Can you work these out from the model? Positions are in its coordinate system, mm. A direction names the side the tool comes from. Give positions to 0.01 mm unless a question says otherwise; leave off trailing zeros. Loops run counter-clockwise (first coordinate to the right, second up) from the corner with the lowest first, then second, coordinate; pieces in that order, holes last. Notation, with made-up numbers: (48, -36.5) - (88, -36.5) arc R11 cw to (88, -28.5) - close; hole circle Ø9 at (-2, -38.75). An arc over 180 degrees is marked (long way). Answer as a JSON object with one key per item and string values. Group by question number.
Item 1: Thinking about a two-plate mould opening in X: for faces 1 (the cylindrical face through (16.3, 7.21, 2.35)), 2 (the flat face through (66.65, 22, 2)), 3 (the flat face through (33, 44.45, 2)), which applies, pulls with the +X half, pulls with the -X half, needs draft (parallel to the pull), parting line crosses it, or undercut?
Item 2: Which directions (+Z, -Z, +X, -X, +Y, -Y) give clear straight access to the entire face, cutting with the end or side of a thin tool? Please do faces 4 (the cylindrical face through (43.9, 25.6, 3.7)), 5 (the cylindrical face through (47.3, 7.21, 2.35)).
Item 3: Will this pin go through, and if not, where does the flat tip stop? pin 1 (18 mm diameter, centred on x = 34.5, y = 23, fed in from +Z).
Item 4: Suppose I cut it at C-C on z = 1.1. Write out the boundary of the cut face in (x, y) (3 decimals).
Item 5: Suppose I cut it at A-A on y = 23. Write out the boundary of the cut face in (x, z), and give its area (3 significant figures).
Item 6: Please list where these lines run through material, in increasing order: L1, parallel to Y at x = 49, z = 1.45; L2, parallel to X at y = 39, z = 3.85; L3, parallel to X at y = 27, z = 4.4.
Item 7: Suppose I cut it at D-D on y = 37. Write out the boundary of the cut face in (x, z), and give its area (3 significant figures).
Item 8: Suppose I cut it at B-B on x = 17.5. Write out the boundary of the cut face in (y, z), and give its area (3 significant figures).
from build123d import *

# Parameters (mm, degrees)
SKETCH1_W            = 66.6496
SKETCH1_H            = 44.45
BOSS_EXTRUDE1_DEPTH  = 4.7625
M3_CLEARANCE_HOLE1_D = 3.2
SKETCH6_R            = 11.1
CUT_EXTRUDE1_DEPTH   = 2.2
SKETCH7_R            = 4.5
CUT_EXTRUDE2_DEPTH   = 81.15321632


with BuildPart() as part:
    # Sketch1 → Boss-Extrude1 (new body)
    with BuildSketch(Plane.XY):
        with Locations((33.3248, 22.225)):
            Rectangle(SKETCH1_W, SKETCH1_H)
    extrude(amount=BOSS_EXTRUDE1_DEPTH)

    # M3 Clearance Hole1 (through all)
    with Locations(Plane.XY.offset(4.7625)):
        with Locations((48.8248, 6.725), (48.8248, 37.725), (17.8248, 6.725), (17.8248, 37.725)):
            Hole(M3_CLEARANCE_HOLE1_D / 2)

    # Sketch6 → Cut-Extrude1 (cut)
    with BuildSketch(Plane.XY.offset(4.7625)):
        with Locations((33.3248, 22.225)):
            Circle(SKETCH6_R)
    extrude(amount=-CUT_EXTRUDE1_DEPTH, mode=Mode.SUBTRACT)

    # Sketch7 → Cut-Extrude2 (cut, through all)
    with BuildSketch(Plane.XY.offset(2.5625)):
        with Locations((33.3248, 22.225)):
            Circle(SKETCH7_R)
    extrude(amount=-CUT_EXTRUDE2_DEPTH, mode=Mode.SUBTRACT)


solid = part.part
Worked out:
{
 "1": {"face 1": "undercut", "face 2": "pulls with the +X half", "face 3": "needs draft"},
 "2": {"face 4": "+Z", "face 5": "+Z, -Z"},
 "3": {"pin 1": "stops at z = 2.56"},
 "4": {"outline": "(0, 0) - (66.65, 0) - (66.65, 44.45) - (0, 44.45) - close; hole circle Ø3.2 at (17.825, 6.725); hole circle Ø3.2 at (17.825, 37.725); hole circle Ø9 at (33.325, 22.225); hole circle Ø3.2 at (48.825, 6.725); hole circle Ø3.2 at (48.825, 37.725)"},
 "5": {"outline": "(0, 0) - (28.89, 0) - (28.89, 2.56) - (22.25, 2.56) - (22.25, 4.76) - (0, 4.76) - close; (37.76, 0) - (66.65, 0) - (66.65, 4.76) - (44.4, 4.76) - (44.4, 2.56) - (37.76, 2.56) - close", "area": "246 mm2"},
 "6": {"L1": "y = 0 to 5.13, 8.32 to 36.13, 39.32 to 44.45", "L2": "x = 0 to 16.86, 18.79 to 47.86, 49.79 to 66.65", "L3": "x = 0 to 23.3, 43.35 to 66.65"},
 "7": {"outline": "(0, 0) - (16.4, 0) - (16.4, 4.76) - (0, 4.76) - close; (19.25, 0) - (47.4, 0) - (47.4, 4.76) - (19.25, 4.76) - close; (50.25, 0) - (66.65, 0) - (66.65, 4.76) - (50.25, 4.76) - close", "area": "290 mm2"},
 "8": {"outline": "(0, 0) - (5.16, 0) - (5.16, 4.76) - (0, 4.76) - close; (8.29, 0) - (36.16, 0) - (36.16, 4.76) - (8.29, 4.76) - close; (39.29, 0) - (44.45, 0) - (44.45, 4.76) - (39.29, 4.76) - close", "area": "182 mm2"}
}
